```python
from build123d import *

# Parameters (mm, degrees)
SKETCH1_R           = 2.5
BOSS_EXTRUDE1_DEPTH = 3
SKETCH2_W           = 12.5
SKETCH2_H           = 9
BOSS_EXTRUDE2_DEPTH = 10
SKETCH3_W           = 2
SKETCH3_H           = 3
CUT_EXTRUDE1_DEPTH  = 9
CUT_EXTRUDE2_DEPTH  = 5
FILLET1_R           = 2
FILLET2_R           = 0.5


with BuildPart() as part:
    # Sketch1 → Boss-Extrude1 (new body)
    with BuildSketch(Plane(origin=(0, 0, 0), x_dir=(1, 0, 0), z_dir=(0, 1, 0))):
        with BuildLine():
            Line((-7.5, -4.5), (8, -4.5))
            ThreePointArc((8, -4.5), (12.5, 0), (8, 4.5))
            Line((8, 4.5), (-7.5, 4.5))
            Line((-7.5, 4.5), (-7.5, -4.5))
        make_face()
        with Locations(Location((8, 0, 0), (0, 0, 270))):
            Circle(SKETCH1_R, mode=Mode.SUBTRACT)
    extrude(amount=BOSS_EXTRUDE1_DEPTH)

    # Sketch2 → Boss-Extrude2 (add)
    with BuildSketch(Plane(origin=(0, 3, 0), x_dir=(1, 0, 0), z_dir=(0, 1, 0))):
        with Locations((-3.25, 0)):
            Rectangle(SKETCH2_W, SKETCH2_H)
    extrude(amount=BOSS_EXTRUDE2_DEPTH)

    # Sketch3 → Cut-Extrude1 (cut)
    with BuildSketch(Plane.XY.offset(4.5)):
        Polygon((-9.5, 3), (-7.5, 3), (-7.933333333, 4), (-7.933333333, 13), (-9.5, 13), align=None)
        Polygon((-7.933333333, 13), (-7.933333333, 4), (-6.647619425, 13), align=None)
        Polygon((-7.5, 0), (-6.2, 0), (-7.5, 3), align=None)
        with Locations((-8.5, 1.5)):
            Rectangle(SKETCH3_W, SKETCH3_H)
        Polygon((3, 13), (-6.647619425, 13), (-0.982644513, 12.190718107), (3, 3), align=None)
    extrude(amount=-CUT_EXTRUDE1_DEPTH, mode=Mode.SUBTRACT)

    # Sketch5 → Cut-Extrude2 (cut)
    with BuildSketch(Plane(origin=(-8.3346666, 1.190666308, 0), x_dir=(0, 0, 1), z_dir=(-0.9899494994718544, 0.14142131556248963, 0))):
        Polygon((0, 10.933541985), (-2.775501763, 9.596930781), (-3.460994088, 6.593592669), (-1.540287274, 4.185102504), (1.540287274, 4.185102504), (3.460994088, 6.593592669), (2.775501763, 9.596930781), align=None)
    extrude(amount=-CUT_EXTRUDE2_DEPTH, mode=Mode.SUBTRACT)

    # Fillet1
    fillet1_edges = [part.edges().sort_by_distance(p)[0] for p in [
        (3, 3, 0),
        (-0.982644513, 12.190718107, 0),
    ]]
    fillet(fillet1_edges, radius=FILLET1_R)

    # Fillet2
    fillet2_edges = [part.edges().sort_by_distance(p)[0] for p in [
        (6.156518848, 3, 4.5),
        (-1.159565612, 11.958901825, 4.5),
        (-1.159565612, 11.958901825, -4.5),
        (3.215410654, 3.328110388, -4.5),
        (3.215410654, 3.328110388, 4.5),
        (12.5, 3, 0),
        (6.156518848, 3, -4.5),
        (-7.066666667, 2, -4.5),
        (-7.933333333, 4, 0),
        (-7.066666667, 2, 4.5),
        (-7.290476379, 8.5, 4.5),
        (-7.290476379, 8.5, -4.5),
        (-6.647619425, 13, 0),
        (-4.368863316, 12.674463509, -4.5),
        (-4.368863316, 12.674463509, 4.5),
        (0.970043929, 7.684514009, 4.5),
        (0.970043929, 7.684514009, -4.5),
    ]]
    fillet(fillet2_edges, radius=FILLET2_R)


solid = part.part
```
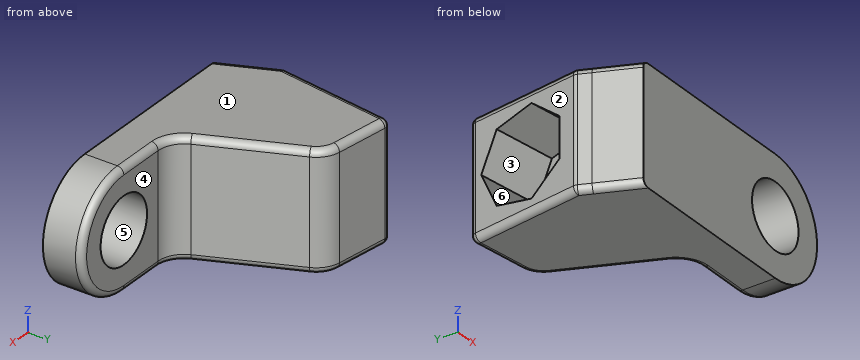
Input: part model. Units: mm. Frame: model coordinates. Face numbers are marked on the shaded views. A direction names the side the tool comes from. Give positions to 0.01 mm unless a question says otherwise; leave off trailing zeros. Loops run counter-clockwise (first coordinate to the right, second up) from the corner with the lowest first, then second, coordinate; pieces in that order, holes last. Notation, with made-up numbers: (69, 38.5) -> (127, 38.5) arc R27 cw to (127, 64.5) -> close; hole circle Ø4 at (-16, 43). An arc over 180 degrees is marked (long way). Use a Markdown table: item, result.
Q1. First-contact query: P1, Ø1, axis at y = 3, z = 2, coming from the +X side; P2, Ø1, axis at y = 11, z = 3, coming from the +X side. Flat tips, straight axial feed; report the tip coordinate or a pass-through.
Entries:
| item | result |
|---|---|
| P1 | stops at x = 12.16 |
| P2 | stops at x = -0.25 |
Q2. Access query for the marked faces 4, 5 and 6. Directions: +Z, -Z, +X, -X, +Y, -Y. A direction counts if a zero-diameter tool reaches every point of the face in a straight line with its end or side. Return the directions, or none.
Entries:
| item | result |
|---|---|
| face 4 | +Z, -Z, +X, +Y |
| face 5 | +Y, -Y |
| face 6 | -X |
Q3. Pull-direction query (Z, two-part tool) for the marked faces 1, 2 and 3; classes: pulls with the +Z half, pulls with the -Z half, needs draft (parallel to the pull), parting line crosses it, or undercut.
Entries:
| item | result |
|---|---|
| face 1 | pulls with the +Z half |
| face 2 | needs draft |
| face 3 | undercut |
Q4. Ray query, probe 1 along X at (y, z) = (1, 0.75); probe 2 along Y at (x, z) = (9, -3); probe 3 along X at (y, z) = (1.6, 0). Return the intervals inside material, ascending. Write a range as from..to.
Entries:
| item | result |
|---|---|
| probe 1 | x = -6.63..5.62, 10.38..12.44 |
| probe 2 | y = 0..3 |
| probe 3 | x = -6.89..5.5, 10.5..12.5 |
Q5. Section query A-A, the plane x = 5.25. Return the cut outline in (y, z), plus the area to 3 significant figures.
Entries:
| item | result |
|---|---|
| outline | (0, -4.5) -> (2.5, -4.5) arc R0.5 ccw to (3, -4) -> (3, 4) arc R0.5 ccw to (2.5, 4.5) -> (0, 4.5) -> close |
| area | 26.9 mm² |
